Could you check a few things on this model? Use its own coordinates, in mm. Face numbers are marked on the shaded views. A direction names the side the tool comes from. Give positions to 0.01 mm unless a question says otherwise; leave off trailing zeros. Order: outer loops, then holes, each group sorted by start corner. A loop starts at its lowest first (then second) coordinate and runs counter-clockwise, first axis right, second up. Notation, with made-up numbers: M 4.5,68.25 L 63.5,68.25 A29 cw 63.5,95.25 Z; hole C 61.25,59 d4. An arc over 180 degrees is marked long. Use a Markdown table: item, result. Add a question column.
Item 1: Suppose I cut it at C-C on y = 3. Write out the boundary of the cut face in (x, z), plus the area to 3 significant figures.
Item 2: Suppose I cut it at A-A on x = 5. Write out the boundary of the cut face in (y, z), plus the area to 4 significant figures.
Item 3: If I drill on L1, parallel to Y at x = 5, z = 0.9; L2, parallel to Z at x = 4, y = 11; L3, parallel to X at y = 18.5, z = -3.5, over which ranges is the centre line in solid material (lowest first)? Write a range as from..to.
Item 4: I'm going to push flat-ended pins straight in: pin 1 Ø1.1 at (y, z) = (15, -3) entering from +X; pin 2 Ø1.3 at (y, z) = (20.5, -1.5) entering from -X; pin 3 Ø1.2 at (y, z) = (29.5, 6) entering from +X; pin 4 Ø1 at (y, z) = (10.5, -1) entering from -X. Where does each tip first touch, or does it pass through?
Item 5: For the marked faces 1, 2, 3, 4 and 5, which set-ups out of +Z, -Z, +X, -X, +Y, -Y let a thin tool reach every point of the face, with its end or its side?
Item 6: Suppose I cut it at D-D on y = 17.5. Write out the boundary of the cut face in (x, z).
Item 7: Suppose I cut it at B-B on z = -2.75. Write out the boundary of the cut face in (x, y).
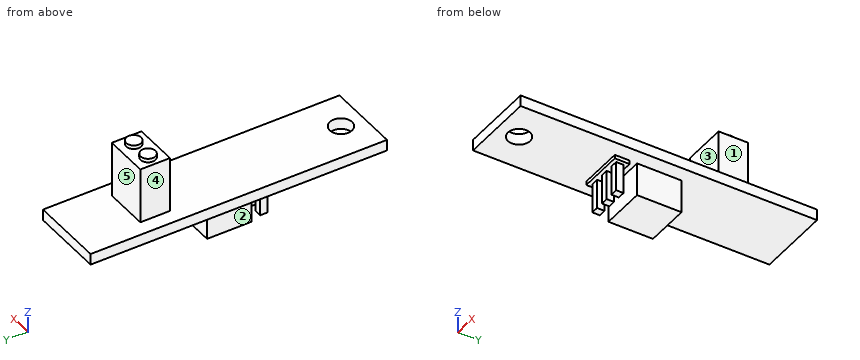
from build123d import *

# Parameters (mm, degrees)
SKETCH_2_W          = 10
SKETCH_2_H          = 40
SKETCH_2_R          = 1.5
EXTRUDE_1_DEPTH     = 1.5
SKETCH_3_W          = 6
SKETCH_3_H          = 4
EXTRUDE_2_DEPTH     = 8
SKETCH_3_3_W        = 6
SKETCH_3_3_H        = 6
EXTRUDE_3_DEPTH     = 6
SKETCH_3_4_W        = 6
SKETCH_3_4_H        = 2
EXTRUDE_4_DEPTH     = 2
SKETCH_4_W          = 1
SKETCH_4_H          = 1
EXTRUDE_5_DEPTH     = 4
SKETCH_5_W          = 6
SKETCH_5_H          = 4
SKETCH_5_R          = 1
CUT_EXTRUDE_1_DEPTH = 0.5


with BuildPart() as part:
    # 草圖2 → 填料-伸長1 (new body)
    with BuildSketch(Plane.XY):
        with Locations((5, 20)):
            Rectangle(SKETCH_2_W, SKETCH_2_H)
        with Locations((5, 3)):
            Circle(SKETCH_2_R, mode=Mode.SUBTRACT)
    extrude(amount=EXTRUDE_1_DEPTH)

    # 草圖3 → 填料-伸長2 (add)
    with BuildSketch(Plane.XY.offset(1.5)):
        with Locations((5, 30)):
            Rectangle(SKETCH_3_W, SKETCH_3_H)
    extrude(amount=EXTRUDE_2_DEPTH)

    # 草圖3<3> → 填料-伸長3 (add)
    with BuildSketch(Plane.XY.offset(1.5)):
        with Locations((5, 20)):
            Rectangle(SKETCH_3_3_W, SKETCH_3_3_H)
    extrude(amount=-EXTRUDE_3_DEPTH)

    # 草圖3<4> → 填料-伸長4 (add)
    with BuildSketch(Plane.XY.offset(1.5)):
        with Locations((5, 15)):
            Rectangle(SKETCH_3_4_W, SKETCH_3_4_H)
    extrude(amount=-EXTRUDE_4_DEPTH)

    # 草圖4 → 填料-伸長5 (add)
    with BuildSketch(Plane(origin=(0, 0, -0.5), x_dir=(-1, 0, 0), z_dir=(0, 0, -1))):
        with Locations((-5, 15)):
            Rectangle(SKETCH_4_W, SKETCH_4_H)
        with Locations((-7, 15)):
            Rectangle(SKETCH_4_W, SKETCH_4_H)
        with Locations((-3, 15)):
            Rectangle(SKETCH_4_W, SKETCH_4_H)
    extrude(amount=EXTRUDE_5_DEPTH)

    # 草圖5 → 除料-伸長1 (cut)
    with BuildSketch(Plane.XY.offset(9.5)):
        with Locations((5, 30)):
            Rectangle(SKETCH_5_W, SKETCH_5_H)
        with Locations((3.5, 30)):
            Circle(SKETCH_5_R, mode=Mode.SUBTRACT)
        with Locations((6.5, 30)):
            Circle(SKETCH_5_R, mode=Mode.SUBTRACT)
    extrude(amount=-CUT_EXTRUDE_1_DEPTH, mode=Mode.SUBTRACT)


solid = part.part
Findings below:
| question | item | result |
|---|---|---|
| 1 | outline | M 0,0 L 3.5,0 L 3.5,1.5 L 0,1.5 Z; M 6.5,0 L 10,0 L 10,1.5 L 6.5,1.5 Z |
| 1 | area | 10.5 mm^2 |
| 2 | outline | M 0,0 L 1.5,0 L 1.5,1.5 L 0,1.5 Z; M 4.5,0 L 14,0 L 14,-0.5 L 14.5,-0.5 L 14.5,-4.5 L 15.5,-4.5 L 15.5,-0.5 L 16,-0.5 L 16,0 L 17,0 L 17,-4.5 L 23,-4.5 L 23,0 L 40,0 L 40,1.5 L 32,1.5 L 32,9 L 28,9 L 28,1.5 L 4.5,1.5 Z |
| 2 | area | 117.5 mm^2 |
| 3 | L1 | y = 0..1.5, 4.5..40 |
| 3 | L2 | z = 0..1.5 |
| 3 | L3 | x = 2..8 |
| 4 | pin 1 | stops at x = 7.5 |
| 4 | pin 2 | stops at x = 2 |
| 4 | pin 3 | stops at x = 8 |
| 4 | pin 4 | passes through |
| 5 | face 1 | +Z, +X, +Y, -Y |
| 5 | face 2 | -Z, -X, +Y, -Y |
| 5 | face 3 | +Z, +X, -X, -Y |
| 5 | face 4 | +Z, -X, +Y, -Y |
| 5 | face 5 | +Z, +X, -X, +Y |
| 6 | outline | M 0,0 L 2,0 L 2,-4.5 L 8,-4.5 L 8,0 L 10,0 L 10,1.5 L 0,1.5 Z |
| 7 | outline | M 2,17 L 8,17 L 8,23 L 2,23 Z; M 2.5,14.5 L 3.5,14.5 L 3.5,15.5 L 2.5,15.5 Z; M 4.5,14.5 L 5.5,14.5 L 5.5,15.5 L 4.5,15.5 Z; M 6.5,14.5 L 7.5,14.5 L 7.5,15.5 L 6.5,15.5 Z |
